Autodesk Inventor part; units mm, degrees
ref_plane "YZ Plane" through (0, 0, 0) normal (1, 0, 0) x (0, 1, 0)
ref_plane "XZ Plane" through (0, 0, 0) normal (0, 1, 0) x (-1, 0, 0)
ref_plane "XY Plane" through (0, 0, 0) normal (0, 0, 1) x (1, 0, 0)
sketch "Sketch1" plane through (0, 0, 0) normal (0, 0, 1) x (1, 0, 0)
  circle A0 centre (0, 0) radius 3
  circle A1 centre (0, 0) radius 5.25
  dimension "d0" = 6
  dimension "d1" = 10.5
extrude "Extrusion1" add sketch "Sketch1" along normal blind 0.8
extrude "Extrusion2" add sketch "Sketch1" along normal blind 25.8 contours A0
thread "Thread1"
sketch "Boceto3" plane through (0, 0, 0) normal (0, 0, -1) x (-1, 0, 0)
  circle A0 centre (0, 0) radius 5.25
extrude "Extrusión3" add sketch "Boceto3" along normal blind 2.5
fillet "Empalme2" radius 2.5 1 edges at (5.25, 0, -2.5)
sketch "Boceto4" plane through (0, 0, -2.5) normal (0, 0, -1) x (-1, 0, 0)
  line L0 (-2.2122, -1.978) -> (-2.8191, 0.9269)
  line L1 (-2.8191, 0.9269) -> (-0.6069, 2.9049)
  line L2 (-0.6069, 2.9049) -> (2.2122, 1.978)
  line L3 (2.2122, 1.978) -> (2.8191, -0.9269)
  line L4 (2.8191, -0.9269) -> (0.6069, -2.9049)
  line L5 (0.6069, -2.9049) -> (-2.2122, -1.978)
  point P0 (0, 0)
  point P1 (0, 0)
  dimension "d12" = 5.14
extrude "Extrusión4" cut sketch "Boceto4" against normal blind 2.5
chamfer "Chaflán1" distance 0.2 angle 45 1 edges at (-3, 0, 25.8)
properties part number "Tornillo Allen cabeza botón M6x25mm"
Can you work these out from the model? Positions are in its coordinate system, mm. A direction names the side the tool comes from. Coordinates: 2 decimals unless noted, no trailing zeros. Loops run counter-clockwise (first coordinate to the right, second up) from the corner with the lowest first, then second, coordinate; pieces in that order, holes last.
1) Thinking about a two-plate mould opening in X: for faces 1 (the flat face through (0, 0, 0)), 2 (the flat face through (2.3, -2.3, 0.8)), 3 (the cylindrical face through (-3, 0, 13)), which applies, pulls with the +X half, pulls with the -X half, needs draft (parallel to the pull), parting line crosses it, or undercut?
2) Imagine slicing it at B-B on z = 13. List the corners of the cut face in (x, y) for me.
3) Which directions (+Z, -Z, +X, -X, +Y, -Y) give clear straight access to the entire face, cutting with the end or side of a thin tool? Please do faces 4 (the flat face through (0, 0, 25.8)), 5 (the flat face through (0.78, -2.45, -1.27)).
4) Imagine slicing it at A-A on y = 0. List the corners of the cut face in (x, z) for me, plus the area to 3 significant figures.
5) For pin 1 (4 mm diameter, centred on x = -2.5, y = 2, fed in from +Z); pin 2 (1.5 mm diameter, centred on x = -1.5, z = 8.5, fed in from +Y); pin 3 (3 mm diameter, centred on y = -4, z = 15, fed in from -X); pin 4 (5 mm diameter, centred on x = -1, z = 9.5, fed in from -Y), each with a flat end and sliding along its axis, tell me the tip position at first contact or that it passes through.
6) I need wall thicknesses on probe 1 along Z at (x, y) = (0.25, 1); probe 2 along Y at (x, z) = (-1.75, 9.5); probe 3 along Z at (x, y) = (-3, 1.25). Which ranges of each line are inside material? Lowest first, please.
Completed:
1. face 1: undercut
1. face 2: needs draft
1. face 3: parting line crosses it
2. outline: circle Ø6 at (0, 0)
3. face 4: +Z, +X, -X, +Y, -Y
3. face 5: -Z
4. outline: (-5.25, 0) arc R2.5 ccw to (-2.75, -2.5) - (-2.63, -2.5) - (-2.63, 0) - (2.63, 0) - (2.63, -2.5) - (2.75, -2.5) arc R2.5 ccw to (5.25, 0) - (5.25, 0.8) - (3, 0.8) - (3, 25.6) - (2.8, 25.8) - (-2.8, 25.8) - (-3, 25.6) - (-3, 0.8) - (-5.25, 0.8) - close
4. area: 169 mm2
5. pin 1: stops at z = 25.8
5. pin 2: stops at y = 2.9
5. pin 3: stops at x = -1.66
5. pin 4: stops at y = -3
6. probe 1: z = 0 to 25.8
6. probe 2: y = -2.44 to 2.44
6. probe 3: z = -2.45 to 0.8
